from build123d import *

# Parameters (mm, degrees)
BOSS_EXTRUDE1_DEPTH     = 0.5
CUT_EXTRUDE1_DEPTH      = 1006.633971904
CUT_EXTRUDE1_DEPTH_BACK = 1006.633971904
SKETCH2_R               = 4


with BuildPart() as part:
    # Sketch1 → Boss-Extrude1 (new, symmetric)
    with BuildSketch(Plane.YZ):
        with BuildLine():
            Line((-152.879110482, 15.875), (-84.862670824, 915.257797566))
            ThreePointArc((-84.862670824, 915.257797566), (0, 993.945), (84.862670824, 915.257797566))
            Line((84.862670824, 915.257797566), (152.879110482, 15.875))
            Line((152.879110482, 15.875), (-152.879110482, 15.875))
        make_face()
    extrude(amount=BOSS_EXTRUDE1_DEPTH, both=True)

    # Sketch2 → Cut-Extrude1 (cut, two sides: drawn at the far end of the back side and taken through both)
    with BuildSketch(Plane.YZ.offset(0.5).offset(-CUT_EXTRUDE1_DEPTH_BACK)):
        with Locations(Location((71.374429386, 695.789702433, 0), (0, 0, 270))):
            Circle(SKETCH2_R)
        with Locations(Location((109.079602796, 197.213409477, 0), (0, 0, 270))):
            Circle(SKETCH2_R)
        with Locations(Location((0, 963.945, 0), (0, 0, 270))):
            Circle(SKETCH2_R)
        with Locations(Location((-71.374429386, 695.789702433, 0), (0, 0, 270))):
            Circle(SKETCH2_R)
        with Locations(Location((-109.079602796, 197.213409477, 0), (0, 0, 270))):
            Circle(SKETCH2_R)
    extrude(amount=CUT_EXTRUDE1_DEPTH + CUT_EXTRUDE1_DEPTH_BACK, mode=Mode.SUBTRACT)


solid = part.part
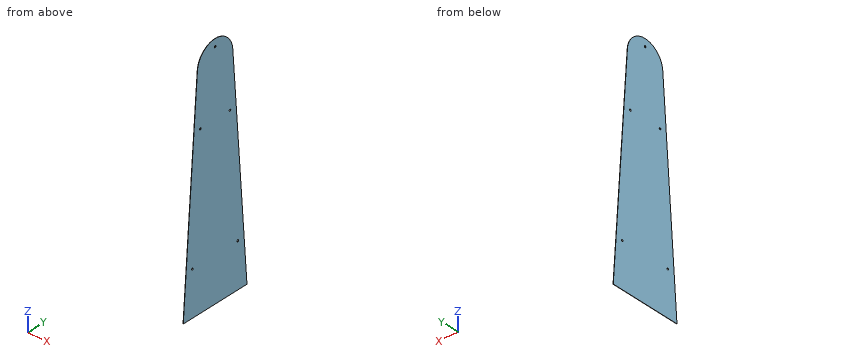
Build history of the part. All positions in model axes, mm. Round coordinates to 2 decimals unless told otherwise and drop trailing zeros. Write each loop counter-clockwise with the first axis right and the second up, starting at its lowest first coordinate (ties: lowest second). Pieces come first, ordered by that corner, then holes. Notation, with made-up numbers: M 23.25,86.5 L 67.25,86.5 A13 ccw 67.25,91.5 Z; hole C 44.5,41 d5. An arc over 180 degrees is marked long. Answer as a JSON object with one key per item and string values. Group by question number.
(1) Cut at A-A (x = -0.2). Give the cut face in (y, z) (3 decimals), and give its area (3 significant figures).
(2) Drill centre lines: L1, parallel to Y at x = -0.1, z = 197; L2, parallel to Z at x = -0.2, y = -50 (3 decimals); L3, parallel to Y at x = -0.2, z = 951. Where is each one in solid material? Low to high.
(3) Cut at B-B (z = 680). Give the cut face in (x, y).
(4) Cut at C-C (y = -126). Give the cut face in (x, z) (3 decimals).
Responses:
{
 "1": {"outline": "M -152.879,15.875 L 152.879,15.875 L 84.863,915.258 A85.105 ccw -84.863,915.258 Z; hole C -109.08,197.213 d8; hole C -71.374,695.79 d8; hole C 0,963.945 d8; hole C 71.374,695.79 d8; hole C 109.08,197.213 d8", "area": "224,000 mm2"},
 "2": {"L1": "y = -139.18 to -113.07, -105.09 to 105.09, 113.07 to 139.18", "L2": "z = 15.875 to 977.708", "L3": "y = -73.93 to 73.93"},
 "3": {"outline": "M -0.5,-102.65 L 0.5,-102.65 L 0.5,102.65 L -0.5,102.65 Z"},
 "4": {"outline": "M -0.5,15.875 L 0.5,15.875 L 0.5,371.298 L -0.5,371.298 Z"}
}
